Verification items for the finished model (mm, model axes). Face numbers are marked on the shaded views. A direction names the side the tool comes from. Coordinates: 2 decimals unless noted, no trailing zeros. Order: outer loops, then holes, each group sorted by start corner. A loop starts at its lowest first (then second) coordinate and runs counter-clockwise, first axis right, second up. Notation, with made-up numbers: M 73,-32 L 126,-32 A29 cw 126,-7 Z; hole C 30.25,18.5 d5. An arc over 180 degrees is marked long. Write item = value, one per line.
```python
from build123d import *

# Parameters (mm, degrees)
FILLET1_R          = 3
FILLET2_R          = 2
FILLET3_R          = 5
SKETCH2_W          = 152
SKETCH2_H          = 13
CUT_EXTRUDE2_DEPTH = 10


with BuildPart() as part:
    # Sketch1 → Revolve1 (revolve)
    with BuildSketch(Plane.XY, mode=Mode.PRIVATE) as revolve1_sk:
        Polygon((-289.147853111, -40.947499885), (335.852146889, -40.947499885), (335.852146889, 27.052500115), (223.852146889, 27.052500115), (223.852146889, 34.052500115), (160.852146889, 34.052500115), (160.852146889, 34.252500115), (22.852146889, 34.252500115), (22.852146889, 44.052500115), (-149.147853111, 44.052500115), (-149.147853111, 56.552500115), (-167.147853111, 56.552500115), (-167.147853111, 44.052500115), (-215.147853111, 44.052500115), (-215.147853111, 34.052500115), (-289.147853111, 34.052500115), align=None)
    revolve(revolve1_sk.sketch.rotate(Axis((-289.147853111, -40.947499885, 0), (1, 0, 0)), 180), axis=Axis((-289.147853111, -40.947499885, 0), (1, 0, 0)))

    # Fillet1
    fillet1_edges = [part.edges().sort_by_distance(p)[0] for p in [
        (-149.147853111, 44.052500115, 0),
    ]]
    fillet(fillet1_edges, radius=FILLET1_R)

    # Fillet2
    fillet2_edges = [part.edges().sort_by_distance(p)[0] for p in [
        (22.852146889, 34.252500115, 0),
    ]]
    fillet(fillet2_edges, radius=FILLET2_R)

    # Fillet3
    fillet3_edges = [part.edges().sort_by_distance(p)[0] for p in [
        (223.852146889, 27.052500115, 0),
    ]]
    fillet(fillet3_edges, radius=FILLET3_R)

    # Sketch2 → Cut-Extrude2 (cut, symmetric)
    with BuildSketch(Plane.XY):
        with Locations((-63.147853111, 37.552500115)):
            Rectangle(SKETCH2_W, SKETCH2_H)
    extrude(amount=CUT_EXTRUDE2_DEPTH, both=True, mode=Mode.SUBTRACT)


solid = part.part
```
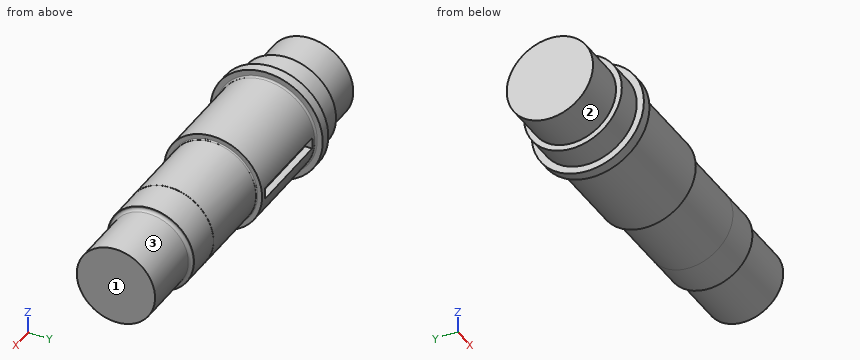
Item 1: Gauge pin test, flat ends, axial feed: pin 1 (10 mm diameter, centred on x = -32.5, y = 40, fed in from +Z); pin 2 (8 mm diameter, centred on x = -194.5, z = -22.5, fed in from +Y); pin 3 (1 mm diameter, centred on x = -168.5, y = 20, fed in from +Z). Record the tip position at first contact, or that the pin passes through.
Report:
pin_1 = 38.17
pin_2 = 42.01
pin_3 = 59.76
Item 2: Scan lines: L1, parallel to X at y = -4.5, z = -64.5; L2, parallel to X at y = -42.5, z = 82; L3, parallel to Y at x = 287, z = 43.5. Record each from-to range of solid material in increasing order. Write a range as from..to.
Report:
L1 = -289.15..223.85
L2 = -215.15..22.85
L3 = -93.21..11.32
Item 3: Tool access check on the marked faces 1, 2 and 3. Record the directions out of +Z, -Z, +X, -X, +Y, -Y that give a thin tool (end or side, any length) a straight path to the whole face; none if there is none.
Report:
face_1 = +Z, -Z, +X, +Y, -Y
face_2 = -X
face_3 = +X
Item 4: Sectioned sample at A-A, the plane x = -10. Enter the section's corners in (y, z), then the cut area to 3 significant figures.
Report:
outline = M 31.05,-10 L 31.05,10 L 43.46,10 A85 ccw long 43.46,-10 Z
area = 22,400 mm^2
Item 5: Sectioned sample at B-B, the plane x = 260. Enter the section's corners in (y, z).
Report:
outline = C -40.95,0 d136
